Answer from the drawing. Dimensions are ordinates in mm from the lowest x, y and z of the part. Give positions to 0.01 mm unless a question says otherwise; leave off trailing zeros. Loops run counter-clockwise (first coordinate to the right, second up) from the corner with the lowest first, then second, coordinate; pieces in that order, holes last. Notation, with made-up numbers: (3, -26.75) -> (9, -26.75) arc R23 cw to (9, 11.25) -> close; hole circle Ø4 at (71.5, 49.5). An arc over 180 degrees is marked (long way). Return JSON: item names as keys, results as strings. Group by question number.
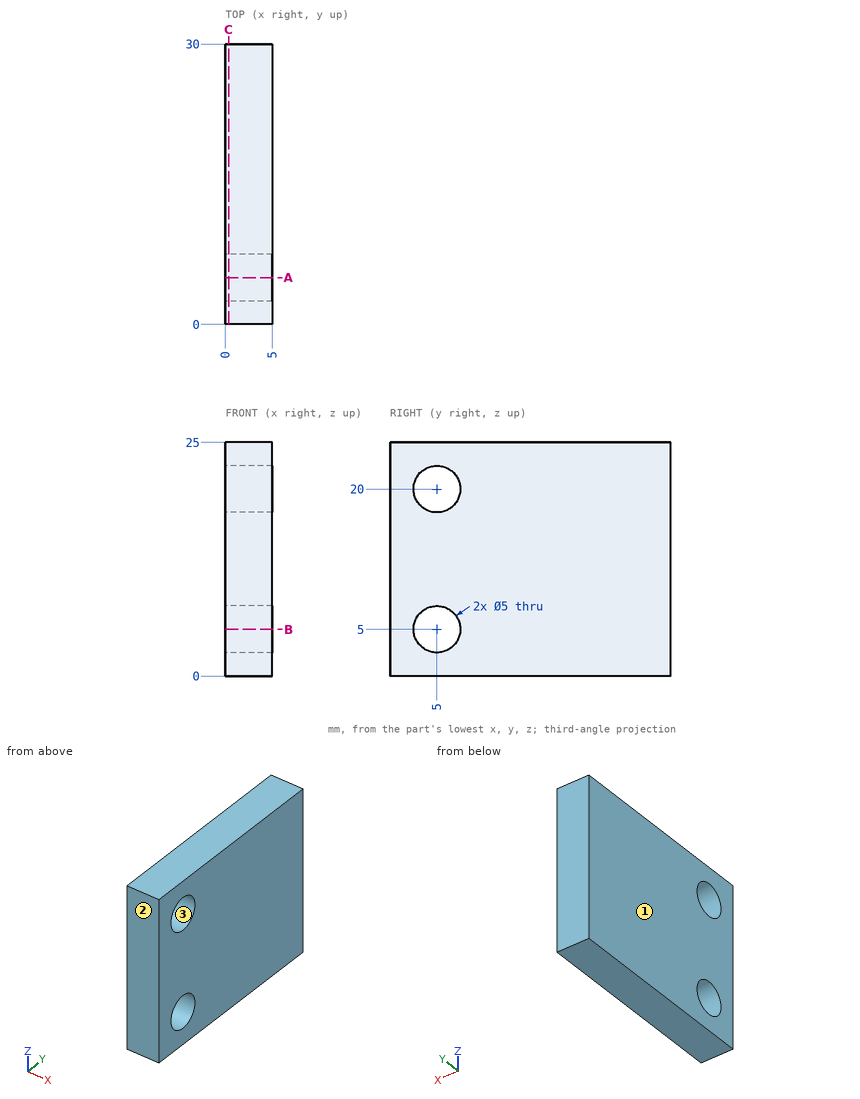
1. Determine the mould class of the marked faces 1, 2 and 3 for opening direction Y: pulls with the +Y half, pulls with the -Y half, needs draft (parallel to the pull), parting line crosses it, or undercut.
2. A flat-ended cylindrical pin translates along its axis: pin 1 Ø4 at (y, z) = (6, 18.5) entering from -X. Find the tip coordinate at first contact, or state that the pin passes through.
3. Section C-C on x = 0.35 is taken. Determine the outline of the cut face in (y, z), then the cut area to 3 significant figures.
4. Section B-B on z = 5 is taken. Determine the outline of the cut face in (x, y), then the cut area to 3 significant figures.
5. Section A-A on y = 5 is taken. Determine the outline of the cut face in (x, z).
6. Straight lines are drawn through the part: line 1 (Z direction, x = 2.15, y = 5); line 2 (Y direction, x = 3.1, z = 5); line 3 (Z direction, x = 2.35, y = 6.5). For each, find the intervals that lie inside material, in ascending order. Write a range as from..to.
Completed:
{
 "1": {"face 1": "needs draft", "face 2": "pulls with the -Y half", "face 3": "undercut"},
 "2": {"pin 1": "stops at x = 0"},
 "3": {"outline": "(0, 0) -> (30, 0) -> (30, 25) -> (0, 25) -> close; hole circle Ø5 at (5, 5); hole circle Ø5 at (5, 20)", "area": "711 mm²"},
 "4": {"outline": "(0, 0) -> (5, 0) -> (5, 2.5) -> (0, 2.5) -> close; (0, 7.5) -> (5, 7.5) -> (5, 30) -> (0, 30) -> close", "area": "125 mm²"},
 "5": {"outline": "(0, 0) -> (5, 0) -> (5, 2.5) -> (0, 2.5) -> close; (0, 7.5) -> (5, 7.5) -> (5, 17.5) -> (0, 17.5) -> close; (0, 22.5) -> (5, 22.5) -> (5, 25) -> (0, 25) -> close"},
 "6": {"line 1": "z = 0..2.5, 7.5..17.5, 22.5..25", "line 2": "y = 0..2.5, 7.5..30", "line 3": "z = 0..3, 7..18, 22..25"}
}
